For this review, use the dimensioned drawing (mm, ordinates from the lowest corner) and the shaded views. A direction names the side the tool comes from. Give positions to 0.01 mm unless a question says otherwise; leave off trailing zeros. Write each loop counter-clockwise with the first axis right and the second up, starting at its lowest first coordinate (ties: lowest second). Pieces come first, ordered by that corner, then holes. Notation, with made-up numbers: M 10,-37 L 36,-37 A17 ccw 36,-13 Z; hole C -21.5,49.25 d6. An arc over 180 degrees is marked long. Use a Markdown table: item, result. Add a question column.
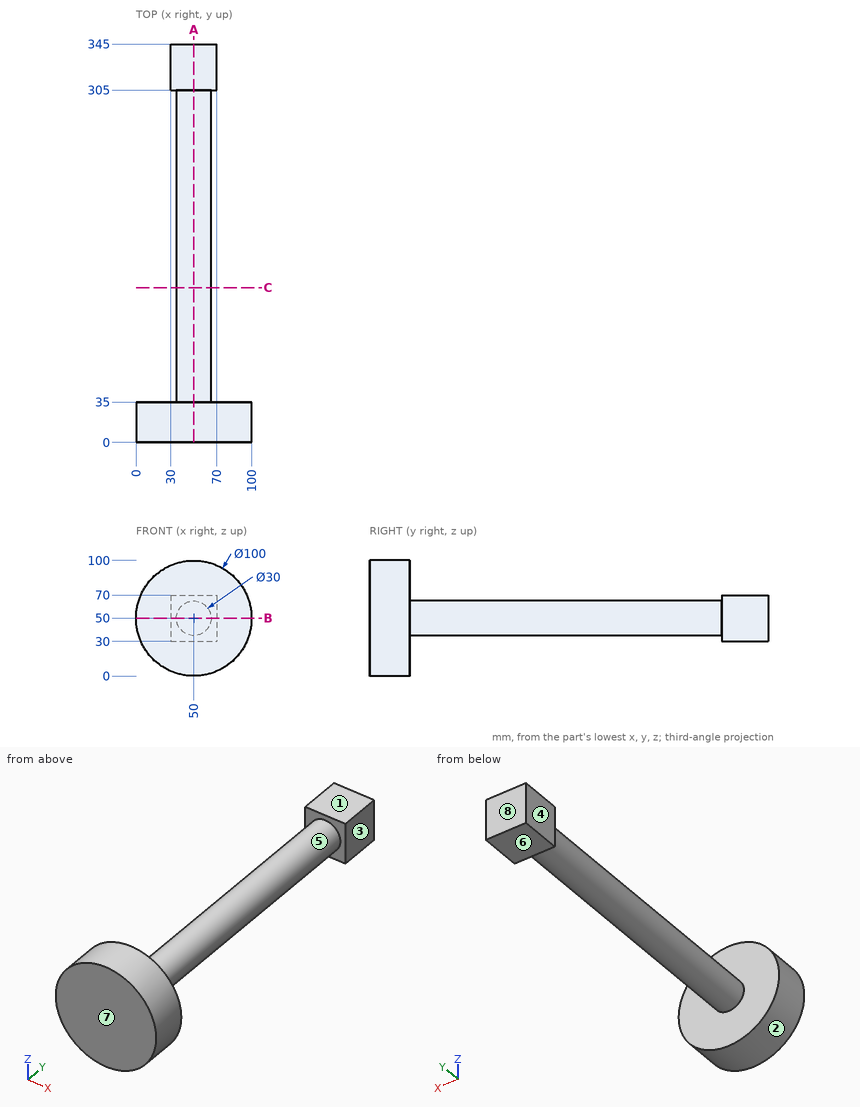
(1) Wall thickness on L1, parallel to Y at x = 35, z = 57; L2, parallel to Y at x = 51.5, z = 20; L3, parallel to Z at x = 39, y = 327.5: over which ranges is each line inside the solid? List them lowest first.
(2) Add section B-B on z = 50. Give the boundary of the cut face in (x, y), then the cut area to 3 significant figures.
(3) The part is to be moulded in two halves that separate along Y. For the marked faces 5, 6, 7 and 8, say which applies: released by +Y, released by -Y, zero draft, split by the parting line, or undercut.
(4) For pin 1 (1.5 mm diameter, centred on y = 208, z = 54, fed in from -X); pin 2 (20 mm diameter, centred on x = 53, y = 315.5, fed in from -Z); pin 3 (4 mm diameter, centred on x = 47, y = 255.5, fed in from +Z), all flat-tipped, find the tip position at first contact; note any pin that passes through.
(5) Add section A-A on x = 50. Give the boundary of the cut face in (y, z).
(6) Machinability: for the marked faces 1, 2, 3 and 4, which of the approach directions +Z, -Z, +X, -X, +Y, -Y give a long, thin tool a straight path to every point of the face, cutting with its end or side? Answer none if there is none.
(7) Add section C-C on y = 134. Give the boundary of the cut face in (x, z), then the cut area to 3 significant figures.
From the geometry:
| question | item | result |
|---|---|---|
| 1 | L1 | y = 0 to 35, 305 to 345 |
| 1 | L2 | y = 0 to 35 |
| 1 | L3 | z = 30 to 70 |
| 2 | outline | M 0,0 L 100,0 L 100,35 L 65,35 L 65,305 L 70,305 L 70,345 L 30,345 L 30,305 L 35,305 L 35,35 L 0,35 Z |
| 2 | area | 13,200 mm^2 |
| 3 | face 5 | undercut |
| 3 | face 6 | zero draft |
| 3 | face 7 | released by -Y |
| 3 | face 8 | released by +Y |
| 4 | pin 1 | stops at x = 35.36 |
| 4 | pin 2 | stops at z = 30 |
| 4 | pin 3 | stops at z = 64.97 |
| 5 | outline | M 0,0 L 35,0 L 35,35 L 305,35 L 305,30 L 345,30 L 345,70 L 305,70 L 305,65 L 35,65 L 35,100 L 0,100 Z |
| 6 | face 1 | +Z, +X, -X, +Y |
| 6 | face 2 | +Y, -Y |
| 6 | face 3 | +Z, -Z, +X, +Y |
| 6 | face 4 | +Z, -Z, -X, +Y |
| 7 | outline | C 50,50 d30 |
| 7 | area | 707 mm^2 |
